Autodesk Inventor part; units mm, degrees
ref_plane "Arbeitsebene2" through (-82.5, -53.5, 0) normal (0, 0, 1) x (1, 0, 0)
ref_plane "YZ Plane" through (0, 0, 0) normal (1, 0, 0) x (0, 1, 0)
ref_plane "XZ Plane" through (0, 0, 0) normal (0, 1, 0) x (-1, 0, 0)
ref_plane "Arbeitsebene1" through (0, 0, 8) normal (0, 0, 1) x (1, 0, 0)
sketch "Skizze1" plane through (0, 0, 8) normal (0, 0, 1) x (1, 0, 0)
  arc A0 (2.5, 0) -> (0, 2.5) centre (0, 0) ccw
  line L0 (-80, 2.5) -> (0, 2.5)
  arc A1 (-80, 2.5) -> (-82.5, 0) centre (-80, 0) ccw
  line L1 (-82.5, -51) -> (-82.5, 0)
  arc A2 (-82.5, -51) -> (-80, -53.5) centre (-80, -51) ccw
  line L2 (0, -53.5) -> (-80, -53.5)
  arc A3 (0, -53.5) -> (2.5, -51) centre (0, -51) ccw
  line L3 (2.5, 0) -> (2.5, -51)
  circle A4 centre (-21, -1) radius 1.25
  circle A5 centre (-79, -1) radius 1.25
  circle A6 centre (-79, -50) radius 1.25
  circle A7 centre (-21, -50) radius 1.25
  line L4 (12.5, 7.5) -> (-177.5, 7.5)
  line L5 (-177.5, 7.5) -> (-177.5, -58.5)
  line L6 (-177.5, -58.5) -> (12.5, -58.5)
  line L7 (12.5, -58.5) -> (12.5, 7.5)
  dimension "d0" = 5
  dimension "d1" = 5
  dimension "d2" = 10
  dimension "d3" = 95
extrude "Extrusion1" add sketch "Skizze1" against normal blind 3 contours L3 A3 L2 A2 L1 A1 L0 A0 | A4 | A5 | A6 | A7 | L7 L6 L5 L4
sketch "Skizze2" plane through (0, 0, 8) normal (0, 0, 1) x (1, 0, 0)
  line L0 (-112.1719, -23.0218) -> (-112.1719, -58.5) construction
  line L1 (12.5, -58.5) -> (-177.5, -58.5) construction
  line L2 (-112.1719, -23.0218) -> (-112.1719, 7.5) construction
  line L3 (-177.5, 7.5) -> (12.5, 7.5) construction
  circle A0 centre (-112.1719, -25.5) radius 12.8913 construction
  circle A1 centre (-112.1719, -25.5) radius 15.2609
  point P0 (0, 0)
  dimension "d6" = 66
extrude "Extrusion2" cut sketch "Skizze2" against normal blind 3
sketch "Skizze3" plane through (0, 0, 5) normal (0, 0, -1) x (-1, 0, 0)
  circle A0 centre (79, -1) radius 1.25
  circle A1 centre (79, -50) radius 1.25
  circle A2 centre (21, -50) radius 1.25
  circle A3 centre (21, -1) radius 1.25
  circle A4 centre (79, -1) radius 3
  circle A5 centre (79, -50) radius 3
  circle A6 centre (21, -1) radius 3
  circle A7 centre (21, -50) radius 3
  point P0 (0, 0)
  dimension "d9" = 6
  dimension "d10" = 6
  dimension "d11" = 6
  dimension "d12" = 6
ref_plane "Arbeitsebene2" through (-82.5, -53.5, 0) normal (0, 0, 1) x (1, 0, 0)
extrude "Extrusion3" add sketch "Skizze3" along normal up to surface (5 mm away) contours A0 | A1 | A2 | A3 | A4 | A5 | A6 | A7
sketch "Skizze4" plane through (-21, -50, 0) normal (0, 0, -1) x (-1, 0, 0)
  circle A0 centre (0, 49) radius 3
  circle A1 centre (58, 49) radius 3
  circle A2 centre (58, 0) radius 3
  circle A3 centre (0, 0) radius 3
  circle A4 centre (0, 49) radius 1
  circle A5 centre (58, 49) radius 1
  circle A6 centre (58, 0) radius 1
  circle A7 centre (0, 0) radius 1
  point P0 (-21, 50)
  dimension "d15" = 2
  dimension "d16" = 2
  dimension "d17" = 2
  dimension "d18" = 2
extrude "Extrusion4" add sketch "Skizze4" along normal blind 3 contours A4 | A5 | A6 | A7
sketch "Skizze8" plane through (0, 0, 5) normal (0, 0, -1) x (-1, 0, 0)
  line L0 (135.1719, -0.5) -> (93.1719, -0.5) construction
  line L1 (93.1719, -0.5) -> (93.1719, -50.5) construction
  line L2 (93.1719, -50.5) -> (135.1719, -50.5) construction
  line L3 (135.1719, -50.5) -> (135.1719, -0.5) construction
  line L4 (135.1719, -0.5) -> (93.1719, -50.5) construction
  line L5 (93.1719, -0.5) -> (135.1719, -50.5) construction
  circle A0 centre (135.1719, -0.5) radius 3.2
  circle A1 centre (135.1719, -50.5) radius 3.2
  circle A2 centre (93.1719, -0.5) radius 3.2
  circle A3 centre (93.1719, -50.5) radius 3.2
  circle A4 centre (112.1719, -25.5) radius 15
  line L6 (144.3139, -20.5597) -> (134.048, -19.05)
  line L7 (134.048, -19.05) -> (128.1099, -2.846)
  line L8 (128.1099, -2.846) -> (116.7369, 0)
  line L9 (116.7369, 0) -> (96.3719, -7.4629)
  line L10 (96.3719, -7.4629) -> (92.1792, -14.1183)
  line L11 (92.1792, -14.1183) -> (87.8515, -27.8062)
  line L12 (87.8515, -27.8062) -> (96.3719, -47.0296)
  line L13 (96.3719, -47.0296) -> (110.7316, -51.5697)
  line L14 (110.7316, -51.5697) -> (144.3139, -44.1668)
  line L15 (144.3139, -44.1668) -> (144.3139, -20.5597)
  line L16 (143.0747, 5.5) -> (85.0747, 5.5)
  line L17 (85.0747, 5.5) -> (85.0747, -56.5)
  line L18 (85.0747, -56.5) -> (143.0747, -56.5)
  line L19 (143.0747, -56.5) -> (143.0747, 5.5)
  line L20 (143.0747, 5.5) -> (85.0747, -56.5) construction
  line L21 (85.0747, 5.5) -> (143.0747, -56.5) construction
  line L22 (200.5, -56.5) -> (195.5, -56.5)
  line L23 (195.5, -56.5) -> (195.5, -51.5)
  line L24 (195.5, -51.5) -> (200.5, -51.5)
  line L25 (200.5, -51.5) -> (200.5, -56.5)
  line L26 (177.5, -58.5) -> (177.5, 7.5)
  line L27 (200.5, 5.5) -> (195.5, 5.5)
  line L28 (195.5, 5.5) -> (195.5, 0.5)
  line L29 (195.5, 0.5) -> (200.5, 0.5)
  line L30 (200.5, 0.5) -> (200.5, 5.5)
  line L31 (4.5, 5.5) -> (9.5, 5.5)
  line L32 (9.5, 5.5) -> (9.5, 0.5)
  line L33 (9.5, 0.5) -> (4.5, 0.5)
  line L34 (4.5, 0.5) -> (4.5, 5.5)
  line L35 (4.5, -56.5) -> (9.5, -56.5)
  line L36 (9.5, -56.5) -> (9.5, -51.5)
  line L37 (9.5, -51.5) -> (4.5, -51.5)
  line L38 (4.5, -51.5) -> (4.5, -56.5)
  point P0 (0, 0)
  point P1 (114.1719, -25.5)
  point P2 (114.0747, -25.5)
  dimension "d24" = 42
  dimension "d25" = 50
  dimension "d26" = 6.4
  dimension "d27" = 6.4
  dimension "d28" = 6.4
  dimension "d29" = 6.4
  dimension "d30" = 2
  dimension "d31" = 0
  dimension "d32" = 58
  dimension "d33" = 62
  dimension "d34" = 0
  dimension "d44" = 5
  dimension "d46" = 5
  dimension "d47" = 5
  dimension "d48" = 5
  dimension "d49" = 5
  dimension "d50" = 5
  dimension "d51" = 5
  dimension "d52" = 5
  dimension "d56" = 0
  dimension "d57" = 23
extrude "Extrusion6" add sketch "Skizze8" along normal blind 24 contours L6 L7 L8 L9 L10 L11 L12 L13 L14 L19 L18 L17 L16 | L22 L23 L24 L25 | L30 L29 L28 L27 | L31 L32 L33 L34 | L38 L37 L36 L35
sketch "Skizze9" plane through (0, 0, -19) normal (0, 0, -1) x (-1, 0, 0)
  line L0 (143.0747, -44.44) -> (110.7316, -51.5697)
  line L1 (110.7316, -51.5697) -> (96.3719, -47.0296)
  line L2 (96.3719, -47.0296) -> (87.8515, -27.8062)
  line L3 (87.8515, -27.8062) -> (92.1792, -14.1183)
  line L4 (92.1792, -14.1183) -> (96.3719, -7.4629)
  line L5 (96.3719, -7.4629) -> (116.7369, 0)
  line L6 (116.7369, 0) -> (128.1099, -2.846)
  line L7 (128.1099, -2.846) -> (134.048, -19.05)
  line L8 (134.048, -19.05) -> (143.0747, -20.3774)
  circle A0 centre (93.1719, -50.5) radius 3.2
  circle A1 centre (93.1719, -0.5) radius 3.2
  circle A2 centre (135.1719, -50.5) radius 3.2
  circle A3 centre (135.1719, -0.5) radius 3.2
  line L9 (143.0747, 5.5) -> (85.0747, 5.5)
  line L10 (85.0747, 5.5) -> (85.0747, -56.5)
  line L11 (85.0747, -56.5) -> (143.0747, -56.5)
  line L12 (143.0747, -20.3774) -> (143.0747, 5.5)
  line L13 (145.3139, -19.696) -> (145.3139, -44.9704)
  line L14 (145.3139, -44.9704) -> (110.6854, -52.6039)
  line L15 (110.6854, -52.6039) -> (95.6405, -47.8471)
  line L16 (95.6405, -47.8471) -> (86.7839, -27.8655)
  line L17 (86.7839, -27.8655) -> (91.2645, -13.6942)
  line L18 (91.2645, -13.6942) -> (95.7076, -6.6413)
  line L19 (95.7076, -6.6413) -> (116.6814, 1.0447)
  line L20 (116.6814, 1.0447) -> (128.8665, -2.0045)
  line L21 (128.8665, -2.0045) -> (134.7822, -18.1472)
  line L22 (134.7822, -18.1472) -> (145.3139, -19.696)
  line L23 (143.0747, -56.5) -> (143.0747, -44.44)
  point P0 (0, 0)
  dimension "d37" = 1
sketch "Skizze15" plane through (-177.5, -58.5, 8) normal (-1, 0, 0) x (0, 0, 1)
  line L0 (0, 66) -> (0, 0)
  line L1 (0, 66) -> (-3, 66)
  line L2 (-3, 0) -> (-3, 66)
  line L3 (0, 0) -> (-3, 0)
  point P0 (-8, 58.5)
extrude "Extrusion10" add sketch "Skizze15" along normal blind 25
ref_plane "Arbeitsebene3" through (-168.3757, -19.6, 1.6) normal (0, 0, 1) x (0, -1, 0)
sketch "Skizze16" plane through (-168.3757, -19.6, 1.6) normal (0, 0, 1) x (0, -1, 0)
  line L0 (-12.5, -14.5) -> (-12.5, 9.5)
  line L1 (-12.5, 9.5) -> (12.5, 9.5)
  line L2 (12.5, 9.5) -> (12.5, -14.5)
  line L3 (12.5, -14.5) -> (-12.5, -14.5)
  circle A0 centre (10.5, -12.5) radius 1.05
  circle A1 centre (10.5, 0) radius 1.05
  circle A2 centre (-10.5, 0) radius 1.05
  circle A3 centre (-10.5, -12.5) radius 1.05
  line L4 (8.7, -9.9) -> (7.48, -9.9)
  line L5 (8.7, -9.1) -> (8.7, -9.9)
  line L6 (7.48, -9.1) -> (8.7, -9.1)
  line L7 (7.48, -9.9) -> (7.48, -9.1)
  point P0 (-19.6, 168.3757)
  point P1 (-3.5315, -12.1603)
extrude "Extrusion11" add sketch "Skizze16" along normal up to surface (3.4 mm away)
sketch "Skizze17" plane through (0, 0, 5) normal (0, 0, -1) x (-1, 0, 0)
  circle A0 centre (168.3757, -9.1) radius 1.05
  circle A1 centre (180.8757, -9.1) radius 1.05
  circle A2 centre (180.8757, -30.1) radius 1.05
  circle A3 centre (168.3757, -30.1) radius 1.05
  line L0 (149.2615, -35.3027) -> (166.5964, -35.3027)
  line L1 (166.5964, -35.3027) -> (166.5964, -5.8969)
  line L2 (166.5964, -5.8969) -> (149.2615, -5.8969)
  line L3 (149.2615, -5.8969) -> (149.2615, -35.3027)
  line L4 (76.1083, -38.9253) -> (91.2151, -38.9253)
  line L5 (91.2151, -38.9253) -> (91.2151, -5.8969)
  line L6 (91.2151, -5.8969) -> (76.1083, -5.8969)
  line L7 (76.1083, -5.8969) -> (76.1083, -38.9253)
  point P0 (0, 0)
extrude "Extrusion12" cut sketch "Skizze17" against normal blind 5
sketch "Skizze18" plane through (0, 0, 8) normal (0, 0, 1) x (1, 0, 0)
  line L0 (-91.2151, -38.9253) -> (-91.2151, -5.8969)
  line L1 (-91.2151, -5.8969) -> (-76.1083, -5.8969)
  line L2 (-76.1083, -5.8969) -> (-76.1083, -38.9253)
  line L3 (-76.1083, -38.9253) -> (-91.2151, -38.9253)
  circle A0 centre (-180.8757, -30.1) radius 1.05
  circle A1 centre (-168.3757, -9.1) radius 1.05
  circle A2 centre (-180.8757, -9.1) radius 1.05
  circle A3 centre (-168.3757, -30.1) radius 1.05
  line L4 (-166.5964, -35.3027) -> (-166.5964, -5.8969)
  line L5 (-166.5964, -5.8969) -> (-149.2615, -5.8969)
  line L6 (-149.2615, -5.8969) -> (-149.2615, -35.3027)
  line L7 (-149.2615, -35.3027) -> (-166.5964, -35.3027)
  circle A4 centre (-112.1719, -25.5) radius 15.2609
  line L8 (12.5, 7.5) -> (-202.5, 7.5)
  line L9 (-202.5, -58.5) -> (-202.5, 7.5)
  line L10 (-202.5, -58.5) -> (12.5, -58.5)
  line L11 (12.5, -58.5) -> (12.5, 7.5)
  line L12 (-91.2151, -5.8969) -> (-149.2615, -5.8969)
  line L13 (-91.2151, -38.9253) -> (-149.2615, -35.3027)
  point P0 (0, 0)
extrude "Extrusion13" cut sketch "Skizze18" against normal blind 1 contours L13 A4 L6 L12 L0 | L13 A4 picked at (-111.0612, -28.7224)
sketch "Skizze19" plane through (0, 0, 5) normal (0, 0, -1) x (-1, 0, 0)
  line L0 (122.2149, -36.9906) -> (149.2615, -35.3027)
  line L1 (149.2615, -35.3027) -> (166.5964, -35.3027)
  line L2 (166.5964, -35.3027) -> (166.5964, -5.8969)
  line L3 (166.5964, -5.8969) -> (76.1083, -5.8969)
  line L4 (76.1083, -5.8969) -> (76.1083, -38.9253)
  line L5 (76.1083, -38.9253) -> (91.2151, -38.9253)
  line L6 (91.2151, -38.9253) -> (103.6356, -38.1501)
  arc A0 (103.6356, -38.1501) -> (122.2149, -36.9906) centre (112.1719, -25.5) ccw
  circle A1 centre (180.8757, -30.1) radius 1.05
  circle A2 centre (168.3757, -9.1) radius 1.05
  circle A3 centre (180.8757, -9.1) radius 1.05
  circle A4 centre (168.3757, -30.1) radius 1.05
  line L7 (-12.5, 7.5) -> (202.5, 7.5)
  line L8 (202.5, -58.5) -> (202.5, 7.5)
  line L9 (202.5, -58.5) -> (-12.5, -58.5)
  line L10 (-12.5, -58.5) -> (-12.5, 7.5)
  circle A5 centre (-4.5, -50.5) radius 1.5
  circle A6 centre (-4.5, 0.5) radius 1.5
  circle A7 centre (194.5, -25.5) radius 1.5
  point P0 (0, 0)
  dimension "d64" = 3
  dimension "d65" = 3
  dimension "d66" = 3
extrude "Extrusion14" cut sketch "Skizze19" against normal through all contours A5 | A6 | A7
properties part number "10_Grundplatte"
Here's how the part is built. I have some questions about the finished solid (model axes, mm). A direction names the side the tool comes from. Round coordinates to 2 decimals unless told otherwise and drop trailing zeros. Order: outer loops, then holes, each group sorted by start corner. A loop starts at its lowest first (then second) coordinate and runs counter-clockwise, first axis right, second up. Notation, with made-up numbers: (-0.75, 25) -> (3.25, 25) arc R25 ccw to (3.25, 50) -> close; hole circle Ø9 at (68.25, 27.5). An arc over 180 degrees is marked (long way). Use CSV: the item, a comma, the result in double quotes.
1. I'm going to push flat-ended pins straight in: P1, Ø1.5, axis at y = 3, z = -2, coming from the -X side; P2, Ø4, axis at y = -53, z = -8.5, coming from the +X side; P3, Ø4, axis at x = -163, y = -14, coming from the +Z side; P4, Ø8, axis at x = -54.5, z = 0.5, coming from the +Y side. Where does each tip first touch, or does it pass through?
Recorded:
P1,"stops at x = -200.5"
P2,"stops at x = -4.5"
P3,"stops at z = 5"
P4,"passes through"
2. I want a section at A-A on z = -13. Give the number of separate pieces and of enclosed holes in the cut face, and give its area (3 significant figures).
Recorded:
separate pieces,"5"
enclosed holes,"4"
area,"1,460 mm2"
3. I want a section at B-B on x = -94. List the corners of the cut face in (y, z) for me.
Recorded:
outline,"(-58.5, 5) -> (-56.5, 5) -> (-56.5, -19) -> (-53.59, -19) -> (-53.59, 5) -> (-47.41, 5) -> (-47.41, -19) -> (-41.68, -19) -> (-41.68, 5) -> (-11.23, 5) -> (-11.23, -19) -> (-3.59, -19) -> (-3.59, 5) -> (2.59, 5) -> (2.59, -19) -> (5.5, -19) -> (5.5, 5) -> (7.5, 5) -> (7.5, 8) -> (-5.9, 8) -> (-5.9, 7) -> (-38.75, 7) -> (-38.75, 8) -> (-58.5, 8) -> close"
4. I want a section at C-C on x = -72.5. List the corners of the cut face in (y, z) for me, and give its area (3 significant figures).
Recorded:
outline,"(-58.5, 5) -> (7.5, 5) -> (7.5, 8) -> (-58.5, 8) -> close"
area,"198 mm2"
5. Which directions (+Z, -Z, +X, -X, +Y, -Y) give clear straight access to the entire face, cutting with the end or side of a thin tool? Please do faces 1 (the face through (-171, -7.1, 3)), 2 (the face through (-9.5, 3, -7)), 3 (the face through (-114, 5.5, -7)), 4 (the face through (-4.5, 3, -7)).
Recorded:
face 1,"-Z, -X, +Y"
face 2,"-Z, +Y, -Y"
face 3,"-Z, +X, -X, +Y"
face 4,"-Z, +X, +Y, -Y"
6. I need wall thicknesses on line 1 along X through (y, z) = (-53, -6.75); line 2 along Y through (x, z) = (-114.5, -1.5); line 3 along Z through (x, y) = (-51.5, -34.5). Which ranges of each line are inside material? Lowest first, please.
Recorded:
line 1,"x = -200.5 to -195.5, -143.07 to -137.17, -133.17 to -95.17, -91.17 to -85.07, -9.5 to -4.5"
line 2,"y = -56.5 to -50.74, -0.82 to 5.5"
line 3,"z = 5 to 8"
7. Thinking about a two-plate mould opening in Y: for faces 5 (the face through (-7, -56.5, -7)), 6 (the face through (-101, -4, -19)), 7 (the face through (-78, -49, 0)), which applies, pulls with the +Y half, pulls with the -Y half, needs draft (parallel to the pull), parting line crosses it, or undercut?
Recorded:
face 5,"pulls with the -Y half"
face 6,"needs draft"
face 7,"undercut"
